CAD build for the part. Positions are in the model's coordinates, mm. Face numbers are marked on the shaded views. A direction names the side the tool comes from. Coordinates: 2 decimals unless noted, no trailing zeros. Write each loop counter-clockwise with the first axis right and the second up, starting at its lowest first coordinate (ties: lowest second). Pieces come first, ordered by that corner, then holes.
```python
from build123d import *

# Parameters (mm, degrees)
F0_W     = 38.1
F0_H     = 38.1
F1_DEPTH = 19.05
F2_DEPTH = 6.35
F4_D     = 6.35
F5_D     = 12.7


with BuildPart() as f1:
    # F0 (on Top) → F1 (new body, symmetric)
    with BuildSketch(Plane.XY):
        with Locations((19.05, 19.05)):
            Rectangle(F0_W, F0_H)
    extrude(amount=F1_DEPTH, both=True)

    # F0 (on Top) → F2 (join, symmetric)
    with BuildSketch(Plane.XY):
        with BuildLine():
            Line((38.1, 38.1), (38.1, 0))
            Line((38.1, 0), (76.2, 0))
            ThreePointArc((76.2, 0), (95.25, 19.05), (76.2, 38.1))
            Line((76.2, 38.1), (38.1, 38.1))
        make_face()
    extrude(amount=F2_DEPTH, both=True)

    # F4 (through all)
    with Locations(Plane.XY.offset(19.05)):
        with Locations((57.15, 25.4), (57.15, 12.7), (76.2, 12.7), (76.2, 25.4)):
            Hole(F4_D / 2)

    # F5 (through all)
    with Locations(Plane.XY.offset(19.05)):
        with Locations((19.05, 19.05)):
            Hole(F5_D / 2)


solid = f1.part
```
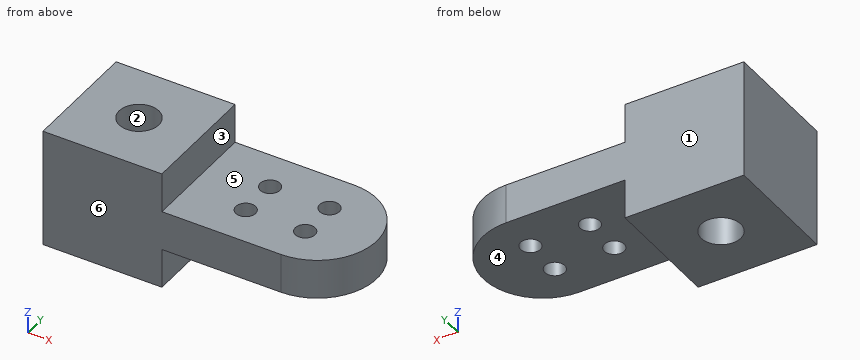
Item 1: Flat gauge pins, fed straight in: pin 1 Ø1.5 at (y, z) = (18, -8.5) entering from +X; pin 2 Ø10 at (x, z) = (78.5, -15) entering from -Y; pin 3 Ø19 at (x, y) = (79, 11) entering from +Z; pin 4 Ø8 at (x, z) = (85.5, 8) entering from -Y. Where does each tip first touch, or does it go through?
Item 2: Saw through at A-A, the plane y = 19.05. Write the cut outline in (x, z).
Item 3: Which spindle directions (+Z, -Z, +X, -X, +Y, -Y) get a long thin tool onto all of the face, cutting with end or side? Do the marked faces 4, 5 and 6. Say none if no direction does.
Item 4: Saw through at D-D, the plane y = 6. Write the cut outline in (x, z).
Item 5: Two-plate mould, pull along Y, no slides. Class the marked faces 1, 2 and 3: +Y half, -Y half, draft (parallel to the pull), parting line (faces both ways), or undercut.
Item 6: Saw through at C-C, the plane z = -11. Write the cut outline in (x, y).
Item 7: Wall check: line 1 along Y through (x, z) = (76, 1); line 2 along Y through (x, z) = (19, -10); line 3 along X through (y, z) = (14.5, 5.5). Give the ranges that are in metal, low to high.
Item 8: Saw through at B-B, the plane z = 5. Write the cut outline in (x, y) (3 decimals), and give its area (3 significant figures).
Working result:
1. pin 1: stops at x = 38.1
1. pin 2: passes through
1. pin 3: stops at z = 6.35
1. pin 4: stops at y = 0.86
2. outline: (0, -19.05) - (12.7, -19.05) - (12.7, 19.05) - (0, 19.05) - close; (25.4, -19.05) - (38.1, -19.05) - (38.1, -6.35) - (95.25, -6.35) - (95.25, 6.35) - (38.1, 6.35) - (38.1, 19.05) - (25.4, 19.05) - close
3. face 4: -Z, +X, +Y, -Y
3. face 5: +Z, +X, +Y, -Y
3. face 6: +Z, -Z, +X, -X, -Y
4. outline: (0, -19.05) - (38.1, -19.05) - (38.1, -6.35) - (90.08, -6.35) - (90.08, 6.35) - (38.1, 6.35) - (38.1, 19.05) - (0, 19.05) - close
5. face 1: +Y half
5. face 2: undercut
5. face 3: draft
6. outline: (0, 0) - (38.1, 0) - (38.1, 38.1) - (0, 38.1) - close; hole circle Ø12.7 at (19.05, 19.05)
7. line 1: y = 0 to 9.53, 15.87 to 22.23, 28.57 to 38.1
7. line 2: y = 0 to 12.7, 25.4 to 38.1
7. line 3: x = 0 to 14.62, 23.48 to 54.53, 59.77 to 73.58, 78.82 to 94.7
8. outline: (0, 0) - (76.2, 0) arc R19.05 ccw to (76.2, 38.1) - (0, 38.1) - close; hole circle Ø12.7 at (19.05, 19.05); hole circle Ø6.35 at (57.15, 12.7); hole circle Ø6.35 at (57.15, 25.4); hole circle Ø6.35 at (76.2, 12.7); hole circle Ø6.35 at (76.2, 25.4)
8. area: 3,220 mm2
